```python
from build123d import *

# Parameters (mm, degrees)
SKETCH_2_W      = 605
SKETCH_2_H      = 75
EXTRUDE_1_DEPTH = 4
EXTRUDE_START   = -4
SKETCH_3_W      = 525
SKETCH_3_H      = 4
EXTRUDE_2_DEPTH = 40


with BuildPart() as part:
    # 스케치2 → 보스-돌출1 (new body)
    with BuildSketch(Plane(origin=(0, 0, 0), x_dir=(1, 0, 0), z_dir=(0, 1, 0))):
        with Locations((302.5, 37.5)):
            Rectangle(SKETCH_2_W, SKETCH_2_H)
    extrude(amount=EXTRUDE_1_DEPTH)

    # 스케치3 → 보스-돌출2 (add)
    with BuildSketch(Plane(origin=(0, 4, 0), x_dir=(1, 0, 0), z_dir=(0, 1, 0)).offset(EXTRUDE_START)):
        with Locations((302.5, 2)):
            Rectangle(SKETCH_3_W, SKETCH_3_H)
        with Locations((302.5, 73)):
            Rectangle(SKETCH_3_W, SKETCH_3_H)
    extrude(amount=EXTRUDE_2_DEPTH)


solid = part.part
```
Source: CAD feature listing. Evaluate the final solid. Frame: model axes, mm. Round coordinates to 2 decimals unless told otherwise and drop trailing zeros. Write each loop counter-clockwise with the first axis right and the second up, starting at its lowest first coordinate (ties: lowest second). Pieces come first, ordered by that corner, then holes. Notation, with made-up numbers: M 40,57 L 64,57 A22 cw 64,74 Z; hole C 14.25,57.25 d1. An arc over 180 degrees is marked long. Use CSV: the item, a comma, the result in double quotes. Start each with the question number.
Q1. First-contact query: P1, Ø2, axis at x = 335.5, y = 5, coming from the +Z side; P2, Ø6, axis at x = 507.5, z = -24, coming from the +Y side; P3, Ø3, axis at y = 29, z = -73, coming from the +X side; P4, Ø3, axis at y = 19.5, z = -72.5, coming from the -X side. Flat tips, straight axial feed; report the tip coordinate or a pass-through.
Q2. Cut plane A-A on y = 15. Output: boundary loops of the cut face in (x, z).
Q3. Pull-direction query (Z, two-part tool) for faces 1 (the face through (298, 20, -75)), 2 (the face through (299, 22, -71)), 3 (the face through (299, 22, -4)), 4 (the face through (298, 0, -38)); classes: +Z half, -Z half, draft (parallel to the pull), parting line (faces both ways), or undercut.
Q4. Cut plane C-C on z = -47. Output: boundary loops of the cut face in (x, y).
Q5. Cut plane B-B on x = 382.5. Output: boundary loops of the cut face in (y, z).
Q6. Line query: line 1 (Z direction, x = 53, y = 32); line 2 (Y direction, x = 161.5, z = -21). Output: solid intervals per line, ascending. Write a range as from..to.
Results found:
1,P1,"z = 0"
1,P2,"y = 4"
1,P3,"x = 565"
1,P4,"x = 40"
2,outline,"M 40,-75 L 565,-75 L 565,-71 L 40,-71 Z; M 40,-4 L 565,-4 L 565,0 L 40,0 Z"
3,face 1,"-Z half"
3,face 2,"undercut"
3,face 3,"undercut"
3,face 4,"draft"
4,outline,"M 0,0 L 605,0 L 605,4 L 0,4 Z"
5,outline,"M 0,-75 L 40,-75 L 40,-71 L 4,-71 L 4,-4 L 40,-4 L 40,0 L 0,0 Z"
6,line 1,"-75..-71, -4..0"
6,line 2,"0..4"
